Drawing for the job (mm, zero at the part's lowest x, y, z). Give positions to 0.01 mm unless a question says otherwise; leave off trailing zeros. Order: outer loops, then holes, each group sorted by start corner. A loop starts at its lowest first (then second) coordinate and runs counter-clockwise, first axis right, second up. Notation, with made-up numbers: (-13, -14) - (10, -14) arc R27 cw to (10, 13) - close; hole circle Ø2 at (-39, -26.75). An arc over 180 degrees is marked (long way). Use a Markdown table: item, result.
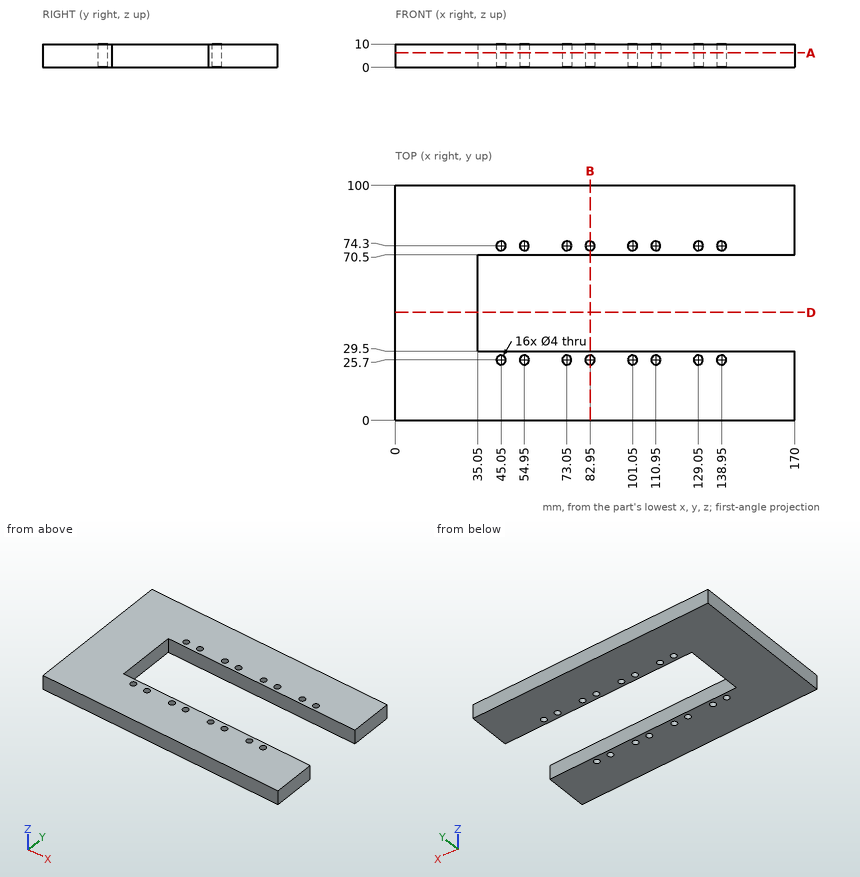
1) Slice it at B-B (x = 82.95). Write the cut outline in (y, z).
Computed:
| item | result |
|---|---|
| outline | (0, 0) - (23.7, 0) - (23.7, 10) - (0, 10) - close; (27.7, 0) - (29.5, 0) - (29.5, 10) - (27.7, 10) - close; (70.5, 0) - (72.3, 0) - (72.3, 10) - (70.5, 10) - close; (76.3, 0) - (100, 0) - (100, 10) - (76.3, 10) - close |
2) Wall check: line 1 (Y direction, x = 111, z = 3); line 2 (Y direction, x = 50.5, z = 6.5); line 3 (X direction, y = 64.5, z = 8). Give the ranges that are in metal, low to high. Write a range as from..to.
Computed:
| item | result |
|---|---|
| line 1 | y = 0..23.7, 27.7..29.5, 70.5..72.3, 76.3..100 |
| line 2 | y = 0..29.5, 70.5..100 |
| line 3 | x = 0..35.05 |
3) Slice it at D-D (y = 46). Write the cut outline in (x, z).
Computed:
| item | result |
|---|---|
| outline | (0, 0) - (35.05, 0) - (35.05, 10) - (0, 10) - close |
4) Slice it at A-A (z = 6.25). State how many separate pieces and enclosed holes the cut face has, and give its area (3 significant figures).
Computed:
| item | result |
|---|---|
| separate pieces | 1 |
| enclosed holes | 16 |
| area | 11,300 mm² |
5) Pin check, flat tips, straight feed: P1, Ø3.5, axis at x = 138.95, y = 74.3, coming from the +Z side; P2, Ø3, axis at y = 55.5, z = 4.5, coming from the +X side. Stop position of each tip, or through.
Computed:
| item | result |
|---|---|
| P1 | passes through |
| P2 | stops at x = 35.05 |
